Design review of the part built by this model. Coordinates are the model's own, in mm. Give positions to 0.01 mm unless a question says otherwise; leave off trailing zeros. Use a Markdown table: item, result. Add a question column.
1. For pin 1 Ø2 at (x, z) = (-0.5, 1) entering from +Y, flat-tipped, find the tip position at first contact; note if it passes through.
2. To check wall thickness, follow line 1 (X direction, y = 0.3, z = 0) (1 decimal); line 2 (X direction, y = 0.35, z = -1). State the ranges of each line that lie inside material, in increasing order.
3. Draft analysis for pull direction X (two halves, no side actions). For faces 1 (the flat face through (0, 0.794, 2)), 2 (the cylindrical face through (-0.207, 0.008, -1.574)), 3 (the cylindrical face through (-0.69, 0.01, 3.1)), state which applies: pulls with the +X half, pulls with the -X half, needs draft (parallel to the pull), parting line crosses it, or undercut.
```python
from build123d import *

# Parameters (mm, degrees)
SKETCH1_W     = 1.5875
SKETCH1_H     = 1.5875
CHAMFER1_SIZE = 0.254


with BuildPart() as part:
    # Sketch1 → Revolve1 (revolve)
    with BuildSketch(Plane.XY):
        with Locations((2.38125, 0)):
            Rectangle(SKETCH1_W, SKETCH1_H)
    revolve(axis=Axis((0, 0, 0), (0, 1, 0)))

    # Chamfer1
    chamfer1_edges = [part.edges().sort_by_distance(p)[0] for p in [
        (-1.5875, -0.79375, 0),
        (-3.175, -0.79375, 0),
        (-3.175, 0.79375, 0),
        (-1.5875, 0.79375, 0),
    ]]
    chamfer(chamfer1_edges, length=CHAMFER1_SIZE)


solid = part.part
```
Taken from the geometry:
| question | item | result |
|---|---|---|
| 1 | pin 1 | stops at y = 0.79 |
| 2 | line 1 | x = -3.2 to -1.6, 1.6 to 3.2 |
| 2 | line 2 | x = -3.01 to -1.23, 1.23 to 3.01 |
| 3 | face 1 | needs draft |
| 3 | face 2 | undercut |
| 3 | face 3 | parting line crosses it |
